Drawing for the job (mm, zero at the part's lowest x, y, z). Coordinates: 2 decimals unless noted, no trailing zeros. Order: outer loops, then holes, each group sorted by start corner. A loop starts at its lowest first (then second) coordinate and runs counter-clockwise, first axis right, second up. Notation, with made-up numbers: M 3,48 L 31,48 A28 cw 31,83 Z; hole C 11,-9 d6. An arc over 180 degrees is marked long. Write item = value, one per line. Start each with the question number.
Q1. Drill centre lines: probe 1 along Y at (x, z) = (83, 2.9); probe 2 along Y at (x, z) = (80, 2.85); probe 3 along X at (y, z) = (26, 3.4). Where is each one in solid material? Low to high.
Q2. Band-saw the part on B-B on z = 0.95. Write the cut outline in (x, y), plus the area to 3 significant figures.
Q3. Band-saw the part on C-C on x = 55. Write the cut outline in (y, z), plus the area to 3 significant figures.
Q4. Band-saw the part on D-D on y = 68.5. Write the cut outline in (x, z), plus the area to 3 significant figures.
Q5. Band-saw the part on A-A on y = 20. Write the cut outline in (x, z).
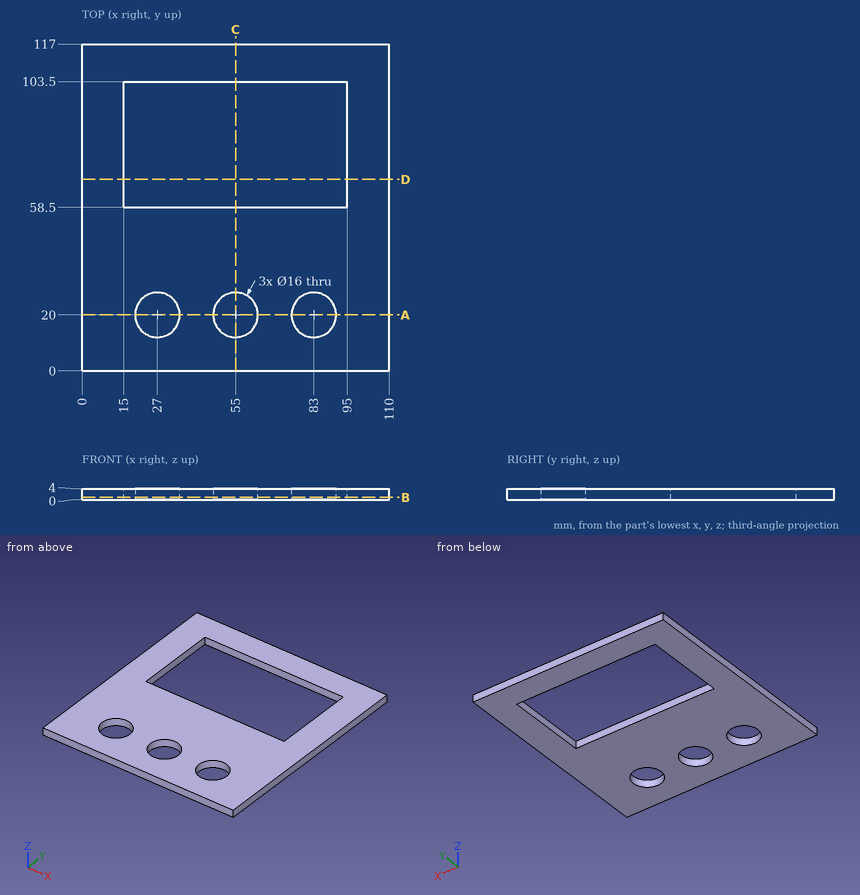
Recorded:
q1.probe_1 = 0 to 12, 28 to 58.5, 103.5 to 117
q1.probe_2 = 0 to 12.58, 27.42 to 58.5, 103.5 to 117
q1.probe_3 = 0 to 21.71, 32.29 to 49.71, 60.29 to 77.71, 88.29 to 110
q2.outline = M 0,0 L 110,0 L 110,117 L 0,117 Z; hole M 15,58.5 L 95,58.5 L 95,103.5 L 15,103.5 Z; hole C 27,20 d16; hole C 55,20 d16; hole C 83,20 d16
q2.area = 8,670 mm2
q3.outline = M 0,0 L 12,0 L 12,4 L 0,4 Z; M 28,0 L 58.5,0 L 58.5,4 L 28,4 Z; M 103.5,0 L 117,0 L 117,4 L 103.5,4 Z
q3.area = 224 mm2
q4.outline = M 0,0 L 15,0 L 15,4 L 0,4 Z; M 95,0 L 110,0 L 110,4 L 95,4 Z
q4.area = 120 mm2
q5.outline = M 0,0 L 19,0 L 19,4 L 0,4 Z; M 35,0 L 47,0 L 47,4 L 35,4 Z; M 63,0 L 75,0 L 75,4 L 63,4 Z; M 91,0 L 110,0 L 110,4 L 91,4 Z
